Build history of the part. All positions in model axes, mm. A direction names the side the tool comes from. Round coordinates to 2 decimals unless told otherwise and drop trailing zeros. Write each loop counter-clockwise with the first axis right and the second up, starting at its lowest first coordinate (ties: lowest second). Pieces come first, ordered by that corner, then holes. Notation, with made-up numbers: (81.5, -5) -> (135.5, -5) arc R14 ccw to (135.5, 1) -> close; hole circle Ø9 at (86.5, -29). An arc over 180 degrees is marked (long way). Return JSON: item names as keys, results as strings.
Autodesk Inventor part; units mm, degrees
ref_plane "YZ Plane" through (0, 0, 0) normal (1, 0, 0) x (0, 1, 0)
ref_plane "XZ Plane" through (0, 0, 0) normal (0, 1, 0) x (-1, 0, 0)
ref_plane "XY Plane" through (0, 0, 0) normal (0, 0, 1) x (1, 0, 0)
sketch "Эскиз1" plane through (0, 0, 0) normal (1, 0, 0) x (0, 1, 0)
  circle A0 centre (0, 0) radius 8.5
  circle A1 centre (0, 0) radius 22.5
  dimension "d0" = 17
  dimension "d1" = 45
extrude "Выдавливание1" add sketch "Эскиз1" along normal blind 20
sketch "Эскиз2" plane through (20, 0, 0) normal (1, 0, 0) x (0, 0, -1)
  circle A0 centre (0, 0) radius 9.5
  dimension "d4" = 19
extrude "Выдавливание2" cut sketch "Эскиз2" against normal blind 6
sketch "Эскиз3" plane through (0, 0, 0) normal (-1, 0, 0) x (0, 0, 1)
  circle A0 centre (0, 0) radius 9.5
  dimension "d7" = 19
extrude "Выдавливание3" cut sketch "Эскиз3" against normal blind 6
sketch "Эскиз4" plane through (0, 0, 0) normal (-1, 0, 0) x (0, 0, 1)
  line L0 (0, 0) -> (-20.5063, 0) construction
  line L1 (-25, -34) -> (25, -34)
  line L2 (25, -34) -> (25, -14)
  line L3 (25, -14) -> (-25, -14)
  line L4 (-25, -14) -> (-25, -34)
  line L5 (0, 0) -> (0, -5.1582) construction
  line L6 (-25, 34) -> (25, 34)
  line L7 (25, 34) -> (25, 14)
  line L8 (25, 14) -> (-25, 14)
  line L9 (-25, 14) -> (-25, 34)
  line L10 (7.5, -14) -> (-7.5, -14)
  line L11 (-7.5, -14) -> (-7.5, -12)
  line L12 (-7.5, -12) -> (7.5, -12)
  line L13 (7.5, -12) -> (7.5, -14)
  line L14 (7.5, 14) -> (-7.5, 14)
  line L15 (-7.5, 14) -> (-7.5, 12)
  line L16 (-7.5, 12) -> (7.5, 12)
  line L17 (7.5, 12) -> (7.5, 14)
  dimension "d10" = 20
  dimension "d11" = 50
  dimension "d12" = 14
  dimension "d18" = 2
  dimension "d19" = 15
extrude "Выдавливание4" cut sketch "Эскиз4" against normal blind 50
sketch "Эскиз5" plane through (0, -14, -17.6139) normal (0, -1, 0) x (1, 0, 0)
  line L0 (0, 25.1139) -> (20, 25.1139)
  line L1 (10, 25.1139) -> (10, 12.2228) construction
  circle A0 centre (10, 30.6139) radius 1.75
  line L2 (0, 17.6139) -> (23.1932, 17.6139) construction
  circle A1 centre (10, 4.6139) radius 1.75
  dimension "d20" = 3.5
  dimension "d21" = 13
extrude "Выдавливание5" cut sketch "Эскиз5" against normal through all
properties part number "04-04-Кулак"
Q1. Saw through at A-A on x = 10. List the corners of the cut face in (y, z).
Verdict:
{"outline": "(-14, -17.61) arc R22.5 ccw to (14, -17.61) -> (14, -14.75) -> (-14, -14.75) -> close; (-14, -11.25) -> (14, -11.25) -> (14, -7.5) -> (12, -7.5) -> (12, 7.5) -> (14, 7.5) -> (14, 11.25) -> (-14, 11.25) -> (-14, 7.5) -> (-12, 7.5) -> (-12, -7.5) -> (-14, -7.5) -> close; (-14, 14.75) -> (14, 14.75) -> (14, 17.61) arc R22.5 ccw to (-14, 17.61) -> close; hole circle Ø17 at (0, 0)"}
Q2. Wall check: L1, parallel to Y at x = 16.2, z = 0; L2, parallel to Z at x = 10, y = -4.5; L3, parallel to Z at x = 10, y = -5.75. Give the ranges that are in metal, low to high.
Verdict:
{"L1": "y = -12 to -9.5, 9.5 to 12", "L2": "z = -22.05 to -14.75, -11.25 to -7.21, 7.21 to 11.25, 14.75 to 22.05", "L3": "z = -21.75 to -14.75, -11.25 to -6.26, 6.26 to 11.25, 14.75 to 21.75"}
Q3. Two-plate mould, pull along Y, no slides. Class faces 1 (the flat face through (8, -14, 13)), 2 (the flat face through (6, -8.4, -2.2)), 3 (the flat face through (0, -10, 0)): +Y half, -Y half, draft (parallel to the pull), parting line (faces both ways), or undercut.
Verdict:
{"face 1": "-Y half", "face 2": "undercut", "face 3": "draft"}
Q4. 3-axis set-ups, long thin cutter, end or side, ignore diameter. For faces 4 (the cylindrical face through (17.04, -8.43, -4.38)), 5 (the flat face through (10, -13, 7.5)), 6 (the flat face through (10, 12, 0)): which of +Z, -Z, +X, -X, +Y, -Y reach the whole face in a straight line?
Verdict:
{"face 4": "+X", "face 5": "+X, -X, -Y", "face 6": "+X, -X, +Y"}
Q5. Saw through at C-C on z = -13. List the corners of the cut face in (x, y), then the cut area to 3 significant figures.
Verdict:
{"outline": "(0, -14) -> (8.25, -14) -> (8.25, 14) -> (0, 14) -> close; (11.75, -14) -> (20, -14) -> (20, 14) -> (11.75, 14) -> close", "area": "462 mm²"}
Q6. Pin check, flat tips, straight feed: pin 1 Ø3 at (x, z) = (12.5, 4.5) entering from -Y; pin 2 Ø1 at (x, y) = (7.5, 13) entering from +Z; pin 3 Ø8 at (x, y) = (4.5, 5) entering from +Z. Stop position of each tip, or through.
Verdict:
{"pin 1": "stops at y = -12", "pin 2": "stops at z = 18.71", "pin 3": "stops at z = 22.48"}
Q7. Saw through at D-D on y = 8. List the corners of the cut face in (x, z), then the cut area to 3 significant figures.
Verdict:
{"outline": "(0, -21.03) -> (20, -21.03) -> (20, -5.12) -> (14, -5.12) -> (14, -2.87) -> (6, -2.87) -> (6, -5.12) -> (0, -5.12) -> close; (0, 5.12) -> (6, 5.12) -> (6, 2.87) -> (14, 2.87) -> (14, 5.12) -> (20, 5.12) -> (20, 21.03) -> (0, 21.03) -> close; hole circle Ø3.5 at (10, -13); hole circle Ø3.5 at (10, 13)", "area": "653 mm²"}
Q8. Saw through at B-B on y = 0. List the corners of the cut face in (x, z).
Verdict:
{"outline": "(0, -22.5) -> (20, -22.5) -> (20, -9.5) -> (14, -9.5) -> (14, -8.5) -> (6, -8.5) -> (6, -9.5) -> (0, -9.5) -> close; (0, 9.5) -> (6, 9.5) -> (6, 8.5) -> (14, 8.5) -> (14, 9.5) -> (20, 9.5) -> (20, 22.5) -> (0, 22.5) -> close; hole circle Ø3.5 at (10, -13); hole circle Ø3.5 at (10, 13)"}
